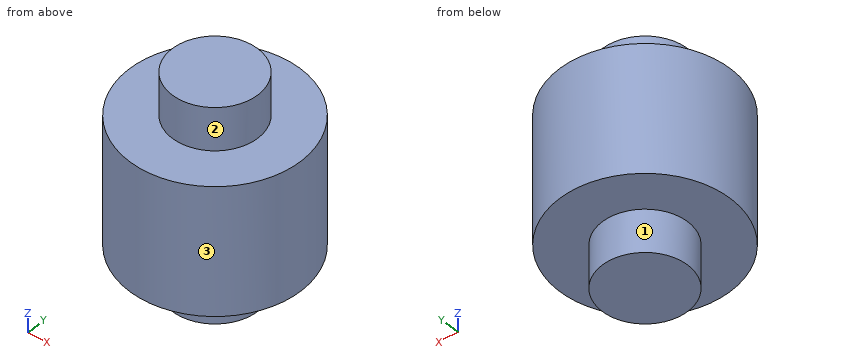
```python
from build123d import *

# Parameters (mm, degrees)
SKETCH_1_R      = 10
EXTRUDE_1_DEPTH = 15
SKETCH_2_R      = 5
EXTRUDE_2_DEPTH = 5


with BuildPart() as part:
    # 스케치1 → 보스-돌출1 (new body)
    with BuildSketch(Plane.XY):
        Circle(SKETCH_1_R)
    extrude(amount=EXTRUDE_1_DEPTH)

    # 스케치2 → 보스-돌출2 (add)
    with BuildSketch(Plane.XY.offset(15)):
        Circle(SKETCH_2_R)
    extrude_2 = extrude(amount=EXTRUDE_2_DEPTH)

    # 대칭 복사1: 보스-돌출2 across plane
    add(extrude_2.mirror(Plane(origin=(0, 0, 7.5), x_dir=(1, 0, 0), z_dir=(0, 0, -1))))


solid = part.part
```
Part model, mm, in its own coordinate system. Face numbers are marked on the shaded views. A direction names the side the tool comes from. Round coordinates to 2 decimals unless told otherwise and drop trailing zeros. Loops run counter-clockwise (first coordinate to the right, second up) from the corner with the lowest first, then second, coordinate; pieces in that order, holes last. Notation, with made-up numbers: (86.5, 56) -> (142.5, 56) arc R20 ccw to (142.5, 63) -> close; hole circle Ø4 at (9.25, -11.75). An arc over 180 degrees is marked (long way). Use a Markdown table: item, result.
1) Probe line 1 (Z direction, x = -1, y = 5); line 2 (Y direction, x = 4.75, z = 12); line 3 (X direction, y = 0.25, z = 18.25). List the from-to ranges inside material, lowest first. Write a range as [from, to].
The answers:
| item | result |
|---|---|
| line 1 | z = [0, 15] |
| line 2 | y = [-8.8, 8.8] |
| line 3 | x = [-4.99, 4.99] |
2) Cut at D-D, the plane x = 8. List the corners of the cut face in (y, z), and give its area (3 significant figures).
The answers:
| item | result |
|---|---|
| outline | (-6, 0) -> (6, 0) -> (6, 15) -> (-6, 15) -> close |
| area | 180 mm2 |
3) Cut at C-C, the plane z = 14. List the corners of the cut face in (x, y).
The answers:
| item | result |
|---|---|
| outline | circle Ø20 at (0, 0) |
4) Cut at A-A, the plane x = 0. List the corners of the cut face in (y, z).
The answers:
| item | result |
|---|---|
| outline | (-10, 0) -> (-5, 0) -> (-5, -5) -> (5, -5) -> (5, 0) -> (10, 0) -> (10, 15) -> (5, 15) -> (5, 20) -> (-5, 20) -> (-5, 15) -> (-10, 15) -> close |
5) Drop flat-ended pins along their axis: pin 1 Ø1 at (x, y) = (5, 3.5) entering from +Z; pin 2 Ø6 at (x, z) = (-6.5, 2) entering from -Y; pin 3 Ø4 at (x, z) = (-7, 4.5) entering from -Y. Give the stop position or say it passes through.
The answers:
| item | result |
|---|---|
| pin 1 | stops at z = 15 |
| pin 2 | stops at y = -9.37 |
| pin 3 | stops at y = -8.66 |
6) Tool access for the marked faces 1, 2 and 3: list every direction of +Z, -Z, +X, -X, +Y, -Y with a clear straight run to the whole face (end or side of a thin tool).
The answers:
| item | result |
|---|---|
| face 1 | -Z |
| face 2 | +Z |
| face 3 | +Z, -Z |
